Could you check a few things on this model? Use its own coordinates, in mm. Give positions to 0.01 mm unless a question says otherwise; leave off trailing zeros. Order: outer loops, then holes, each group sorted by start corner. A loop starts at its lowest first (then second) coordinate and runs counter-clockwise, first axis right, second up. Notation, with made-up numbers: (-21, -33.75) - (-10, -33.75) arc R18 ccw to (-10, -2.75) - close; hole circle Ø3 at (80, -2.75). An arc over 180 degrees is marked (long way). Put each result on its own line as item: value.
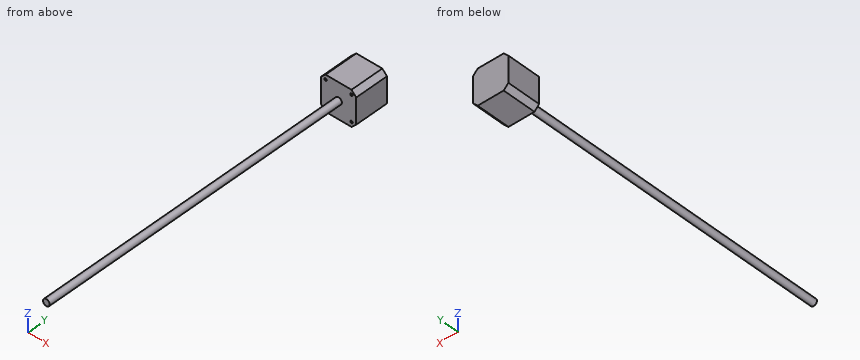
from build123d import *

# Parameters (mm, degrees)
SKETCH_1_R          = 4
EXTRUDE_1_DEPTH     = 380
SKETCH_5_W          = 42.3
SKETCH_5_H          = 42.3
EXTRUDE_5_DEPTH     = 40
SKETCH_7_OUTSIDE_W  = 129.148
SKETCH_7_OUTSIDE_H  = 129.148
CUT_EXTRUDE_1_DEPTH = 422.063706581
SKETCH_8_R          = 1.5
CUT_EXTRUDE_2_DEPTH = 4


with BuildPart() as part:
    # 草图1 → 凸台-拉伸1 (new body)
    with BuildSketch(Plane(origin=(0, 0, 0), x_dir=(1, 0, 0), z_dir=(0, 1, 0))):
        with Locations(Location((0, 0, 0), (0, 0, 270))):
            Circle(SKETCH_1_R)
    extrude(amount=EXTRUDE_1_DEPTH)

    # 草图5 → 凸台-拉伸5 (add)
    with BuildSketch(Plane(origin=(0, 380, 0), x_dir=(1, 0, 0), z_dir=(0, 1, 0))):
        Rectangle(SKETCH_5_W, SKETCH_5_H)
    extrude(amount=EXTRUDE_5_DEPTH)

    # 草图7 outside → 切除-拉伸1 (cut, through all)
    with BuildSketch(Plane(origin=(0, 420, 0), x_dir=(1, 0, 0), z_dir=(0, 1, 0))):
        Rectangle(SKETCH_7_OUTSIDE_W, SKETCH_7_OUTSIDE_H)
        Polygon((-15.5, 21.15), (-21.15, 15.5), (-21.15, -15.5), (-15.5, -21.15), (15.5, -21.15), (21.15, -15.5), (21.15, 15.5), (15.5, 21.15), align=None, mode=Mode.SUBTRACT)
    extrude(amount=-CUT_EXTRUDE_1_DEPTH, mode=Mode.SUBTRACT)

    # 草图8 → 切除-拉伸2 (cut)
    with BuildSketch(Plane.XZ.offset(-380)):
        with Locations(Location((-15.5, 15.5, 0), (0, 0, 270))):
            Circle(SKETCH_8_R)
        with Locations(Location((15.5, 15.5, 0), (0, 0, 270))):
            Circle(SKETCH_8_R)
        with Locations(Location((15.5, -15.5, 0), (0, 0, 270))):
            Circle(SKETCH_8_R)
        with Locations(Location((-15.5, -15.5, 0), (0, 0, 270))):
            Circle(SKETCH_8_R)
    extrude(amount=-CUT_EXTRUDE_2_DEPTH, mode=Mode.SUBTRACT)


solid = part.part
1) Suppose I cut it at B-B, the plane x = 0. List the corners of the cut face in (y, z) for me, and give its area (3 significant figures).
Filled in:
outline: (0, -4) - (380, -4) - (380, -21.15) - (420, -21.15) - (420, 21.15) - (380, 21.15) - (380, 4) - (0, 4) - close
area: 4,730 mm^2
2) If I drill on line 1 (X direction, y = 382, z = -15.5); line 2 (Y direction, x = -14.5, z = -9.5), over which ranges is the centre line in solid material (lowest first)? Write a range as [from, to].
Filled in:
line 1: x = [-21.15, -17], [-14, 14], [17, 21.15]
line 2: y = [380, 420]
3) I'm going to push flat-ended pins straight in: pin 1 (0.9 mm diameter, centred on x = -15, z = 15.5, fed in from -Y); pin 2 (3 mm diameter, centred on x = 6.5, y = 301.5, fed in from +Z); pin 3 (4 mm diameter, centred on x = 15.5, z = -15.5, fed in from -Y); pin 4 (6 mm diameter, centred on x = -1.5, y = 138.5, fed in from +Z). Where does each tip first touch, or does it pass through?
Filled in:
pin 1: stops at y = 384
pin 2: passes through
pin 3: stops at y = 380
pin 4: stops at z = 4
4) Suppose I cut it at C-C, the plane y = 143. List the corners of the cut face in (x, z) for me, and give its area (3 significant figures).
Filled in:
outline: circle Ø8 at (0, 0)
area: 50.3 mm^2
5) Suppose I cut it at A-A, the plane z = 0. List the corners of the cut face in (x, y) for me.
Filled in:
outline: (-21.15, 380) - (-4, 380) - (-4, 0) - (4, 0) - (4, 380) - (21.15, 380) - (21.15, 420) - (-21.15, 420) - close
